from build123d import *

# Parameters (mm, degrees)
MODEL_R             = 0.7834936
MODEL_R_2           = 1.229367
EXTRUDE_1_DEPTH     = 10.3
MODEL_3_W           = 10.5
MODEL_3_H           = 3
EXTRUDE_2_DEPTH     = 8.3
MODEL_4_R           = 6.5
EXTRUDE_3_DEPTH     = 3
SKETCH_2_W          = 28.6
SKETCH_2_H          = 4
EXTRUDE_4_DEPTH     = 1.6
SKETCH_3_W          = 10.5
SKETCH_3_H          = 5.089019843
CUT_EXTRUDE_1_DEPTH = 5.6
MODEL_5_R           = 1.229367
EXTRUDE_5_DEPTH     = 26
MODEL_6_R           = 0.7834936
EXTRUDE_6_DEPTH     = 3
SKETCH_4_R          = 1.229367
EXTRUDE_7_DEPTH     = 3
SKETCH_4_3_R        = 1.229367
CUT_EXTRUDE_2_DEPTH = 8
CHAMFER_1_SIZE      = 3
CUT_EXTRUDE_3_DEPTH = 30


with BuildPart() as part:
    # Model → Extrude 1 (new body)
    with BuildSketch(Plane.XY):
        with BuildLine():
            Line((-28.162112801, 27.669809042), (-37.212112801, 27.669809042))
            Line((-37.212112801, 27.669809042), (-37.212112801, -0.330212606))
            ThreePointArc((-37.212112801, -0.330212606), (-22.912101977, -14.630201782), (-8.612112801, -0.330190958))
            Line((-8.612112801, -0.330190958), (-8.612112801, 27.669809042))
            Line((-8.612112801, 27.669809042), (-17.662112801, 27.669809042))
            Line((-17.662112801, 27.669809042), (-17.662112801, 24.669809042))
            Line((-17.662112801, 24.669809042), (-16.932112801, 24.669809042))
            ThreePointArc((-16.932112801, 24.669809042), (-15.87145263, 24.230469214), (-15.432112801, 23.169809042))
            Line((-15.432112801, 23.169809042), (-15.432112801, -0.330190958))
            ThreePointArc((-15.432112801, -0.330190958), (-22.912112801, -7.810190958), (-30.392112801, -0.330190958))
            Line((-30.392112801, -0.330190958), (-30.392112801, 23.169809042))
            ThreePointArc((-30.392112801, 23.169809042), (-29.952772973, 24.230469214), (-28.892112801, 24.669809042))
            Line((-28.892112801, 24.669809042), (-28.162112801, 24.669809042))
            Line((-28.162112801, 24.669809042), (-28.162112801, 27.669809042))
        make_face()
        with Locations((-33.392112801, -0.330190958)):
            Circle(MODEL_R, mode=Mode.SUBTRACT)
        with Locations((-12.432112801, -0.330190958)):
            Circle(MODEL_R, mode=Mode.SUBTRACT)
        with Locations((-33.392112801, 24.669809042)):
            Circle(MODEL_R, mode=Mode.SUBTRACT)
        with Locations((-12.432112801, 24.669809042)):
            Circle(MODEL_R, mode=Mode.SUBTRACT)
        Polygon((-37.212112801, 31.669809042), (-37.212112801, 27.669809042), (-28.162112801, 27.669809042), (-17.662112801, 27.669809042), (-8.612112801, 27.669809042), (-8.612112801, 31.669809042), align=None)
        with Locations((-33.212112801, 29.669809042)):
            Circle(MODEL_R_2, mode=Mode.SUBTRACT)
        with Locations((-22.912112801, 29.669809042)):
            Circle(MODEL_R_2, mode=Mode.SUBTRACT)
        with Locations((-12.612112801, 29.669809042)):
            Circle(MODEL_R_2, mode=Mode.SUBTRACT)
        with Locations((-33.212112801, 29.669809042)):
            Circle(MODEL_R_2)
        with Locations((-22.912112801, 29.669809042)):
            Circle(MODEL_R_2)
        with Locations((-12.612112801, 29.669809042)):
            Circle(MODEL_R_2)
    extrude(amount=EXTRUDE_1_DEPTH)

    # Model_3 → Extrude 2 (add)
    with BuildSketch(Plane.XY):
        with Locations((-22.912112801, 26.169809042)):
            Rectangle(MODEL_3_W, MODEL_3_H)
    extrude(amount=EXTRUDE_2_DEPTH)

    # Model_4 → Extrude 3 (add)
    with BuildSketch(Plane.XY):
        with BuildLine():
            Line((-30.392112801, -0.330190958), (-30.392112801, 23.169809042))
            ThreePointArc((-30.392112801, 23.169809042), (-29.952772973, 24.230469214), (-28.892112801, 24.669809042))
            Line((-28.892112801, 24.669809042), (-16.932112801, 24.669809042))
            ThreePointArc((-16.932112801, 24.669809042), (-15.87145263, 24.230469214), (-15.432112801, 23.169809042))
            Line((-15.432112801, 23.169809042), (-15.432112801, -0.330190958))
            ThreePointArc((-15.432112801, -0.330190958), (-22.912112801, -7.810190958), (-30.392112801, -0.330190958))
        make_face()
        with Locations((-22.912112801, -0.330190958)):
            Circle(MODEL_4_R, mode=Mode.SUBTRACT)
    extrude(amount=EXTRUDE_3_DEPTH)

    # Sketch 2 → Extrude 4 (add)
    with BuildSketch(Plane.XY.offset(10.3)):
        with Locations((-22.912112801, 29.669809042)):
            Rectangle(SKETCH_2_W, SKETCH_2_H)
    extrude(amount=EXTRUDE_4_DEPTH)

    # Sketch 3 → Cut-Extrude 1 (cut)
    with BuildSketch(Plane.XZ.offset(-27.669809042)):
        with Locations((-22.912112801, 10.844509922)):
            Rectangle(SKETCH_3_W, SKETCH_3_H)
    extrude(amount=-CUT_EXTRUDE_1_DEPTH, mode=Mode.SUBTRACT)

    # Model_5 → Extrude 5 (add)
    with BuildSketch(Plane.XY):
        Polygon((-37.212112801, 31.669809042), (-37.212112801, 27.669809042), (-28.162112801, 27.669809042), (-17.662112801, 27.669809042), (-8.612112801, 27.669809042), (-8.612112801, 31.669809042), align=None)
        with Locations((-33.212112801, 29.669809042)):
            Circle(MODEL_5_R, mode=Mode.SUBTRACT)
        with Locations((-22.912112801, 29.669809042)):
            Circle(MODEL_5_R, mode=Mode.SUBTRACT)
        with Locations((-12.612112801, 29.669809042)):
            Circle(MODEL_5_R, mode=Mode.SUBTRACT)
        with Locations((-12.612112801, 29.669809042)):
            Circle(MODEL_5_R)
        with Locations((-22.912112801, 29.669809042)):
            Circle(MODEL_5_R)
        with Locations((-33.212112801, 29.669809042)):
            Circle(MODEL_5_R)
    extrude(amount=-EXTRUDE_5_DEPTH)

    # Model_6 → Extrude 6 (add)
    with BuildSketch(Plane.XY):
        with Locations((-12.432112801, 24.669809042)):
            Circle(MODEL_6_R)
        with Locations((-33.392112801, 24.669809042)):
            Circle(MODEL_6_R)
        with Locations((-33.392112801, -0.330190958)):
            Circle(MODEL_6_R)
        with Locations((-12.432112801, -0.330190958)):
            Circle(MODEL_6_R)
    extrude(amount=EXTRUDE_6_DEPTH)

    # Sketch 4 → Extrude 7 (add)
    with BuildSketch(Plane(origin=(0, 0, -26), x_dir=(-1, 0, 0), z_dir=(0, 0, -1))):
        Polygon((28.912112801, 54.669809042), (16.912112801, 54.669809042), (8.612112801, 31.669809042), (37.212112801, 31.669809042), align=None)
        with Locations((22.912112801, 49.669809042)):
            Circle(SKETCH_4_R, mode=Mode.SUBTRACT)
    extrude(amount=-EXTRUDE_7_DEPTH)

    # Sketch 4_3 → Cut-Extrude 2 (cut)
    with BuildSketch(Plane(origin=(0, 0, -26), x_dir=(-1, 0, 0), z_dir=(0, 0, -1))):
        with Locations((12.612112801, 29.669809042)):
            Circle(SKETCH_4_3_R)
        with Locations((22.912112801, 29.669809042)):
            Circle(SKETCH_4_3_R)
        with Locations((33.212112801, 29.669809042)):
            Circle(SKETCH_4_3_R)
    extrude(amount=-CUT_EXTRUDE_2_DEPTH, mode=Mode.SUBTRACT)

    # Chamfer 1
    chamfer_1_edges = [part.edges().sort_by_distance(p)[0] for p in [
        (-22.912112801, 27.669809042, 0),
    ]]
    chamfer(chamfer_1_edges, length=CHAMFER_1_SIZE)

    # Sketch 5 → Cut-Extrude 3 (cut)
    with BuildSketch(Plane(origin=(-8.612112801, 0, 0), x_dir=(0, 0, -1), z_dir=(1, 0, 0))):
        Polygon((-11.9, 31.669809042), (-11.9, 28.278558322), (-8.50874928, 31.669809042), align=None)
    extrude(amount=-CUT_EXTRUDE_3_DEPTH, mode=Mode.SUBTRACT)


solid = part.part
Can you work these out from the model? Positions are in its coordinate system, mm. A direction names the side the tool comes from. Give positions to 0.01 mm unless a question says otherwise; leave off trailing zeros. Loops run counter-clockwise (first coordinate to the right, second up) from the corner with the lowest first, then second, coordinate; pieces in that order, holes last. Notation, with made-up numbers: (-11, -11) - (-4, -11) arc R16 cw to (-4, 9) - close; hole circle Ø11 at (18, 21). An arc over 180 degrees is marked (long way). Answer as a JSON object with one key per item and string values.
Q1. If we mould it in two halves opening along Y, with no side actions, what happens to faces 1 (the flat face through (-13.07, 29.95, 10.23)), 2 (the flat face through (-23, 38, -26)), 3 (the cylindrical face through (-32.95, 28.47, -22.06))? For each: pulls with the +Y half, pulls with the -Y half, needs draft (parallel to the pull), parting line crosses it, or undercut.
Geometry says:
{"face 1": "pulls with the +Y half", "face 2": "needs draft", "face 3": "undercut"}
Q2. Will these pins go through, and if not, where does the flat tip stop? P1, Ø7, axis at x = -26, z = -11, coming from the -Y side; P2, Ø7.5, axis at x = -23, y = 30, coming from the +Z side; P3, Ø12, axis at x = -31.5, y = 10.5, coming from the -Z side; P4, Ø10, axis at y = 16, z = -8, coming from the +X side.
Geometry says:
{"P1": "y = 27.67", "P2": "z = 8.3", "P3": "z = 0", "P4": "through"}
Q3. If I drill on L1, parallel to X at y = 1, z = 8; L2, parallel to X at y = 24.5, z = 5; L3, parallel to Z at x = -31, y = 9, over which ranges is the centre line in solid material (lowest first)?
Geometry says:
{"L1": "-37.21 to -30.39, -15.43 to -8.61", "L2": "-37.21 to -34.16, -32.63 to -29.59, -16.24 to -13.2, -11.67 to -8.61", "L3": "0 to 10.3"}
Q4. Which directions (+Z, -Z, +X, -X, +Y, -Y) give clear straight access to the entire face, cutting with the end or side of a thin tool? Please do faces 4 (the flat face through (-14, 7, 10.3)), 5 (the flat face through (-12, 25, 3)), 6 (the flat face through (-33, 30, -18)).
Geometry says:
{"face 4": "+Z, +X, -X, -Y", "face 5": "+Z", "face 6": "-Z"}
Q5. Imagine slicing it at D-D on y = -2.5. Write out the boundary of the cut face in (x, z).
Geometry says:
{"outline": "(-37.05, 0) - (-29.04, 0) - (-29.04, 3) - (-30.07, 3) - (-30.07, 10.3) - (-37.05, 10.3) - close; (-16.78, 0) - (-8.78, 0) - (-8.78, 10.3) - (-15.75, 10.3) - (-15.75, 3) - (-16.78, 3) - close"}
Q6. Imagine slicing it at A-A on z = 7.5. Write out the boundary of the cut face in (x, y).
Geometry says:
{"outline": "(-37.21, -0.33) arc R14.3 ccw to (-8.61, -0.33) - (-8.61, 31.67) - (-37.21, 31.67) - close; hole circle Ø1.57 at (-33.39, -0.33); hole circle Ø1.57 at (-33.39, 24.67); hole (-30.39, -0.33) arc R7.48 ccw to (-15.43, -0.33) - (-15.43, 23.17) arc R1.5 ccw to (-16.93, 24.67) - (-28.89, 24.67) arc R1.5 ccw to (-30.39, 23.17) - close; hole circle Ø1.57 at (-12.43, -0.33); hole circle Ø1.57 at (-12.43, 24.67)"}
Q7. Imagine slicing it at B-B on x = -19.25. Write out the boundary of the cut face in (y, z), plus the area to 3 significant figures.
Geometry says:
{"outline": "(-14.15, 0) - (-5.7, 0) - (-5.7, 3) - (-6.85, 3) - (-6.85, 10.3) - (-14.15, 10.3) - close; (5.04, 0) - (24.67, 0) - (27.67, -3) - (27.67, -26) - (54.67, -26) - (54.67, -23) - (31.67, -23) - (31.67, 8.3) - (24.67, 8.3) - (24.67, 3) - (5.04, 3) - close", "area": "373 mm²"}
Q8. Imagine slicing it at C-C on y = 19. Write out the boundary of the cut face in (x, z).
Geometry says:
{"outline": "(-37.21, 0) - (-8.61, 0) - (-8.61, 10.3) - (-15.43, 10.3) - (-15.43, 3) - (-30.39, 3) - (-30.39, 10.3) - (-37.21, 10.3) - close"}
